```python
from build123d import *

# Parameters (mm, degrees)
SKETCH1_R           = 8
BOSS_EXTRUDE1_DEPTH = 14
SKETCH2_R           = 5.25
CUT_EXTRUDE1_DEPTH  = 14
CHAMFER7_SIZE       = 0.3


with BuildPart() as part:
    # Sketch1 → Boss-Extrude1 (new body)
    with BuildSketch(Plane.XY):
        Circle(SKETCH1_R)
    extrude(amount=BOSS_EXTRUDE1_DEPTH)

    # Sketch2 → Cut-Extrude1 (cut)
    with BuildSketch(Plane.XY):
        Circle(SKETCH2_R)
    extrude(amount=CUT_EXTRUDE1_DEPTH, mode=Mode.SUBTRACT)

    # Chamfer7
    chamfer7_edges = [part.edges().sort_by_distance(p)[0] for p in [
        (-8, 0, 0),
        (-8, 0, 14),
        (-5.25, 0, 0),
        (-5.25, 0, 14),
    ]]
    chamfer(chamfer7_edges, length=CHAMFER7_SIZE)


solid = part.part
```
The model under review builds one solid part; all positions refer to its coordinate system, in mm. Round coordinates to 2 decimals unless told otherwise and drop trailing zeros. Loops run counter-clockwise (first coordinate to the right, second up) from the corner with the lowest first, then second, coordinate; pieces in that order, holes last. Notation, with made-up numbers: (34.5, -22.75) -> (82.5, -22.75) arc R5 ccw to (82.5, -15.75) -> close; hole circle Ø8 at (16.5, 78). An arc over 180 degrees is marked (long way). Answer in a Markdown table with one row per item.
1) Consider section A-A, the plane x = 0. Write out the cut boundary in (y, z), plus the area to 3 significant figures.
Taken from the geometry:
| item | result |
|---|---|
| outline | (-8, 0.3) -> (-7.7, 0) -> (-5.55, 0) -> (-5.25, 0.3) -> (-5.25, 13.7) -> (-5.55, 14) -> (-7.7, 14) -> (-8, 13.7) -> close; (5.25, 0.3) -> (5.55, 0) -> (7.7, 0) -> (8, 0.3) -> (8, 13.7) -> (7.7, 14) -> (5.55, 14) -> (5.25, 13.7) -> close |
| area | 76.6 mm² |
2) Draft analysis for pull direction Y (two halves, no side actions). For faces 1 (the cylindrical face through (5, 1.6, 6.9)), 2 (the flat face through (5, -3, 0)), 3 (the cylindrical face through (-1.73, -7.81, 6.91)), state which applies: pulls with the +Y half, pulls with the -Y half, needs draft (parallel to the pull), parting line crosses it, or undercut.
Taken from the geometry:
| item | result |
|---|---|
| face 1 | undercut |
| face 2 | needs draft |
| face 3 | parting line crosses it |
3) For pin 1 Ø6 at (x, z) = (5, 3.5) entering from +Y; pin 2 Ø3 at (x, z) = (-3, 4) entering from +Y; pin 3 Ø1.5 at (y, z) = (4.5, 3) entering from -X, all flat-tipped, find the tip position at first contact; note any pin that passes through.
Taken from the geometry:
| item | result |
|---|---|
| pin 1 | stops at y = 7.75 |
| pin 2 | stops at y = 7.86 |
| pin 3 | stops at x = -7.07 |
4) Consider section C-C, the plane z = 3.25. Write out the cut boundary in (x, y).
Taken from the geometry:
| item | result |
|---|---|
| outline | circle Ø16 at (0, 0); hole circle Ø10.5 at (0, 0) |
5) Wall thickness on line 1 along Y through (x, z) = (0, 10.75); line 2 along Y through (x, z) = (3, 4); line 3 along X through (y, z) = (-1, 7.5): over which ranges is each line inside the solid? List them lowest first.
Taken from the geometry:
| item | result |
|---|---|
| line 1 | y = -8 to -5.25, 5.25 to 8 |
| line 2 | y = -7.42 to -4.31, 4.31 to 7.42 |
| line 3 | x = -7.94 to -5.15, 5.15 to 7.94 |
